CAD build for the part. Positions are in the model's coordinates, mm. A direction names the side the tool comes from. Round coordinates to 2 decimals unless told otherwise and drop trailing zeros. Loops run counter-clockwise (first coordinate to the right, second up) from the corner with the lowest first, then second, coordinate; pieces in that order, holes last. Notation, with made-up numbers: M 88.5,-13 L 141.5,-13 A7 ccw 141.5,-5 Z; hole C -31,50 d10. An arc over 180 degrees is marked long. Use a Markdown table: item, result. Add a question column.
(1) Flat gauge pins, fed straight in: P1, Ø20.5, axis at y = -8.5, z = -99.5, coming from the -X side; P2, Ø20.5, axis at x = 5.5, z = -107, coming from the -Y side; P3, Ø5, axis at y = -2, z = -92, coming from the +X side. Where does each tip first touch, or does it go through?
(2) Wall check: L1, parallel to X at y = 13, z = -61.5; L2, parallel to X at y = 17, z = -99.5; L3, parallel to Y at x = 13.5, z = -42.5. Give the ranges that are in metal, low to high.
(3) Two-plate mould, pull along X, no slides. Class faces 6 (the face through (6, -18, -114.3)), 7 (the face through (-20.781, -1, -101)), 8 (the face through (0, -17.323, -100)): released by +X, released by -X, zero draft, split by the parting line, or undercut.
(4) Band-saw the part on C-C, the plane x = -5.5. Write the cut outline in (y, z), and give its area (3 significant figures).
(5) Which spindle directions (+Z, -Z, +X, -X, +Y, -Y) get a long thin tool onto all of the face, cutting with end or side? Do faces 1 (the face through (0, -19, -86.36)), 2 (the face through (26.08, -1.42, -83.75)), 3 (the face through (-25.93, -1.42, -83.75)), 4 (the face through (0, 17.864, -100)), 5 (the face through (0, 18.371, -101)). Say none if no direction does.
(6) Band-saw the part on D-D, the plane z = -36.5. Write the cut outline in (x, y), and give its area (3 significant figures).
(7) Band-saw the part on A-A, the plane z = -94. Write the cut outline in (x, y).
(8) Band-saw the part on B-B, the plane y = -14. Write the cut outline in (x, z).
from build123d import *

# Parameters (mm, degrees)
F0_W     = 62.0293021202
F0_H     = 59.1503232718
F1_DEPTH = 88.9
F2_W     = 40.0586724281
F2_H     = 35.1866781712
F3_DEPTH = 76.2
F4_SIZE  = 5.08
F5_SIZE  = 10.16
F6_T     = 2.54
F7_DEPTH = 25.4


# Not quite as in the source:
# - a shell that OpenCascade refuses in one call is made with other operations: the cavity is built on its own and cut out


with BuildPart() as f1:
    # F0 (on Top) → F1 (new body)
    with BuildSketch(Plane.XY):
        with Locations((0.0738501549, -1.0445043445)):
            Rectangle(F0_W, F0_H)
    extrude(amount=-F1_DEPTH)

    # F2 (on face) → F3 (cut, symmetric)
    with BuildSketch(Plane(origin=(0, 0, -88.9), x_dir=(1, 0, 0), z_dir=(0, 0, -1))):
        with Locations((-0.360891223, -0.2706944942)):
            Rectangle(F2_W, F2_H)
    extrude(amount=F3_DEPTH, both=True, mode=Mode.SUBTRACT)

    # F4
    f4_edges = [f1.edges().sort_by_distance(p)[0] for p in [
        (-30.940801, 28.530657, -44.45),
        (31.088501, 28.530657, -44.45),
        (31.088501, -30.619666, -44.45),
        (-30.940801, -30.619666, -44.45),
    ]]
    chamfer(f4_edges, length=F4_SIZE)

    # F5 (call 1 of 4: OpenCascade refuses the feature's edges together)
    f5_edges = [f1.edges().sort_by_distance(p)[0] for p in [
        (0.07385, -30.619666, -88.9),
    ]]
    chamfer(f5_edges, length=F5_SIZE)

    # F5#2 (call 2 of 4)
    f5_2_edges = [f1.edges().sort_by_distance(p)[0] for p in [
        (0.07385, 28.530657, -88.9),
    ]]
    chamfer(f5_2_edges, length=F5_SIZE)

    # F5#3 (call 3 of 4)
    f5_3_edges = [f1.edges().sort_by_distance(p)[0] for p in [
        (31.088501, -1.044504, -88.9),
    ]]
    chamfer(f5_3_edges, length=F5_SIZE)

    # F5#4 (call 4 of 4)
    f5_4_edges = [f1.edges().sort_by_distance(p)[0] for p in [
        (-30.940801, -1.044504, -88.9),
    ]]
    chamfer(f5_4_edges, length=F5_SIZE)

    # F6: shell of thickness 2.54, made by hand


with BuildPart() as f6_core1:
    # F6_t2: copy of F1
    add(f1.part)

    # the walls: a layer under each face that stays
    f6_faces = [f6_core1.faces().sort_by_distance(p)[0] for p in [
        (0.0738501549, 23.4506572914, -83.82),
        (-17.8015650395, -17.6860714609, -88.9),
        (-25.8608009052, -1.0445043445, -83.82),
        (26.008501215, -1.0445043445, -83.82),
        (-28.4008009052, 25.9906572914, -40.64),
        (28.548501215, 25.9906572914, -40.64),
        (0.0738501549, 28.5306572914, -39.37),
        (0.0738501549, -25.5396659803, -83.82),
        (-30.9408009052, -1.0445043445, -39.37),
        (-28.4008009052, -28.0796659803, -40.64),
        (28.548501215, -28.0796659803, -40.64),
        (31.088501215, -1.0445043445, -39.37),
        (0.0738501549, -1.0445043445, 0),
        (0.0738501549, -30.6196659803, -39.37),
    ]]
    thicken(f6_faces, amount=-F6_T, mode=Mode.SUBTRACT)


with BuildPart() as f1_1:
    add(f1.part)

    # what is left inside the walls is the cavity
    f6_cavity = [f6_core1.part.solids().sort_by_distance(p)[0] for p in [
        (0.07385, 25.965257, -52.638598),
    ]]
    add(f6_cavity, mode=Mode.SUBTRACT)

    # F7 (add): a face of the model
    f7_faces = [f1_1.faces().sort_by_distance(p)[0] for p in [
        (0.0738501549, 18.3136708028, -88.9),
    ]]
    extrude(f7_faces, amount=F7_DEPTH)


solid = f1_1.part
Return value:
| question | item | result |
|---|---|---|
| 1 | P1 | x = -20.78 |
| 1 | P2 | y = -20.46 |
| 1 | P3 | x = 20.93 |
| 2 | L1 | -30.94 to -28.4, 28.55 to 31.09 |
| 2 | L2 | -20.78 to -20.39, 19.67 to 20.93 |
| 2 | L3 | -30.62 to -28.08, 25.99 to 28.53 |
| 3 | face 6 | zero draft |
| 3 | face 7 | released by -X |
| 3 | face 8 | undercut |
| 4 | outline | M -30.62,-78.74 L -20.46,-88.9 L -20.46,-114.3 L -17.32,-114.3 L -17.32,-86.36 L -19.41,-86.36 L -28.08,-77.69 L -28.08,-2.54 L 25.99,-2.54 L 25.99,-77.69 L 17.86,-85.81 L 17.86,-114.3 L 18.37,-114.3 L 18.37,-88.9 L 28.53,-78.74 L 28.53,0 L -30.62,0 Z |
| 4 | area | 701 mm^2 |
| 5 | face 1 | none |
| 5 | face 2 | -Z, +X, +Y, -Y |
| 5 | face 3 | -Z, -X, +Y, -Y |
| 5 | face 4 | -Z |
| 5 | face 5 | -Z, +X, -X, +Y |
| 6 | outline | M -30.94,-25.54 L -25.86,-30.62 L 26.01,-30.62 L 31.09,-25.54 L 31.09,23.45 L 26.01,28.53 L -25.86,28.53 L -30.94,23.45 Z; hole M -28.4,-24.49 L -24.81,-28.08 L 24.96,-28.08 L 28.55,-24.49 L 28.55,22.4 L 24.96,25.99 L -24.81,25.99 L -28.4,22.4 Z |
| 6 | area | 564 mm^2 |
| 7 | outline | M -20.78,-20.46 L 20.93,-20.46 L 20.93,18.37 L -20.78,18.37 Z; hole M -20.39,-17.32 L 19.67,-17.32 L 19.67,17.86 L -20.39,17.86 Z |
| 8 | outline | M -30.94,-78.74 L -20.78,-88.9 L -20.78,-114.3 L -20.39,-114.3 L -20.39,-85.7 L -28.4,-77.69 L -28.4,-2.54 L 28.55,-2.54 L 28.55,-77.69 L 19.88,-86.36 L 19.67,-86.36 L 19.67,-114.3 L 20.93,-114.3 L 20.93,-88.9 L 31.09,-78.74 L 31.09,0 L -30.94,0 Z |
